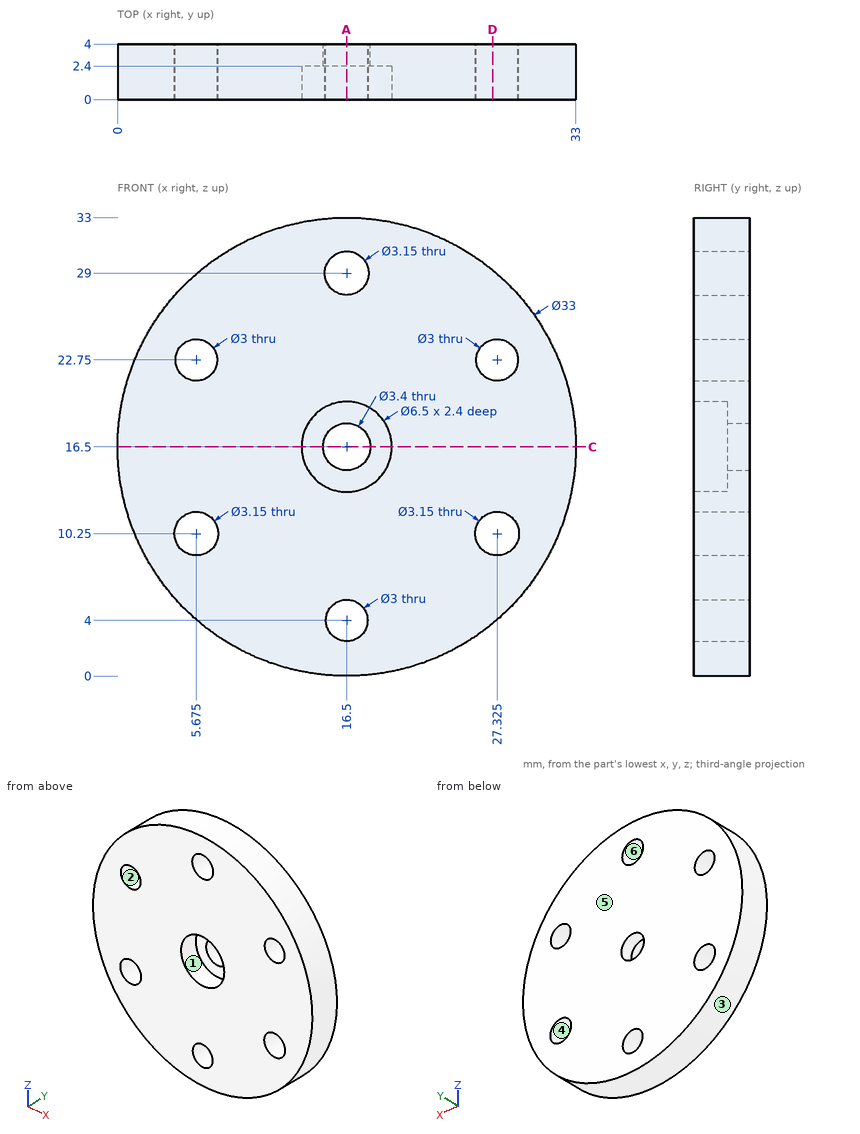
Here's the drawing with two shaded views (mm, measured from the low corner). I have some questions. A direction names the side the tool comes from. Coordinates: 2 decimals unless noted, no trailing zeros. Write each loop counter-clockwise with the first axis right and the second up, starting at its lowest first coordinate (ties: lowest second). Pieces come first, ordered by that corner, then holes. Notation, with made-up numbers: M 3.5,14 L 19.5,14 A24 ccw 19.5,41 Z; hole C 57.5,-11 d8. An arc over 180 degrees is marked long. Use one line per item in the form item = value.
Q1. If we section it at C-C (z = 16.5): Write out the boundary of the cut face in (x, y), then the cut area to 3 significant figures.
Model answer:
outline = M 0,0 L 13.25,0 L 13.25,2.4 L 14.8,2.4 L 14.8,4 L 0,4 Z; M 18.2,2.4 L 19.75,2.4 L 19.75,0 L 33,0 L 33,4 L 18.2,4 Z
area = 111 mm^2
Q2. If we section it at A-A (x = 16.5): State how many separate pieces and enclosed holes the cut face has.
Model answer:
separate_pieces = 4
enclosed_holes = 0
Q3. I need wall thicknesses on line 1 along Z through (x, y) = (6.5, 3) (1 decimal); line 2 along X through (y, z) = (1.65, 22.75) (1 decimal); line 3 along X through (y, z) = (1.05, 29) (1 decimal). Which ranges of each line are inside material? Lowest first, please. Write a range as from..to.
Model answer:
line_1 = 3.4..8.9, 11.6..21.5, 24..29.6
line_2 = 1.2..4.2, 7.2..25.8, 28.8..31.8
line_3 = 5.7..14.9, 18.1..27.3
Q4. We'd pull the mould along Z, two halves only. Please class the marked faces 3, 4, 5 and 6: +Z half, -Z half, draft (parallel to the pull), parting line (faces both ways), or undercut.
Model answer:
face_3 = parting line
face_4 = undercut
face_5 = draft
face_6 = undercut
Q5. For the marked faces 1 and 2, which set-ups out of +Z, -Z, +X, -X, +Y, -Y let a thin tool reach every point of the face, with its end or its side?
Model answer:
face_1 = -Y
face_2 = +Y, -Y
Q6. If we section it at D-D (x = 27): Write out the boundary of the cut face in (y, z).
Model answer:
outline = M 0,3.77 L 4,3.77 L 4,8.71 L 0,8.71 Z; M 0,11.79 L 4,11.79 L 4,21.29 L 0,21.29 Z; M 0,24.21 L 4,24.21 L 4,29.23 L 0,29.23 Z
Q7. For P1, Ø1.5, axis at y = 2.5, z = 21.5, coming from the -X side; P2, Ø1, axis at x = 26, y = 1, coming from the -Z side; P3, Ø5.5, axis at x = 16.5, z = 16.5, coming from the -Y side; P4, Ø1.9, axis at x = 16.5, z = 29, coming from the +Y side, each with a flat end and sliding along its axis, tell me the tip position at first contact or that it passes through.
Model answer:
P1 = 0.56
P2 = 2.67
P3 = 2.4
P4 = through
